Print and shaded views of the part. All mm, measured from the part's lowest x, y and z. A direction names the side the tool comes from. Coordinates: 2 decimals unless noted, no trailing zeros. Loops run counter-clockwise (first coordinate to the right, second up) from the corner with the lowest first, then second, coordinate; pieces in that order, holes last. Notation, with made-up numbers: M 45.5,59 L 68.5,59 A22 ccw 68.5,88 Z; hole C 73,-1 d8. An arc over 180 degrees is marked long. Answer as a JSON object with one key per item and string values. Group by question number.
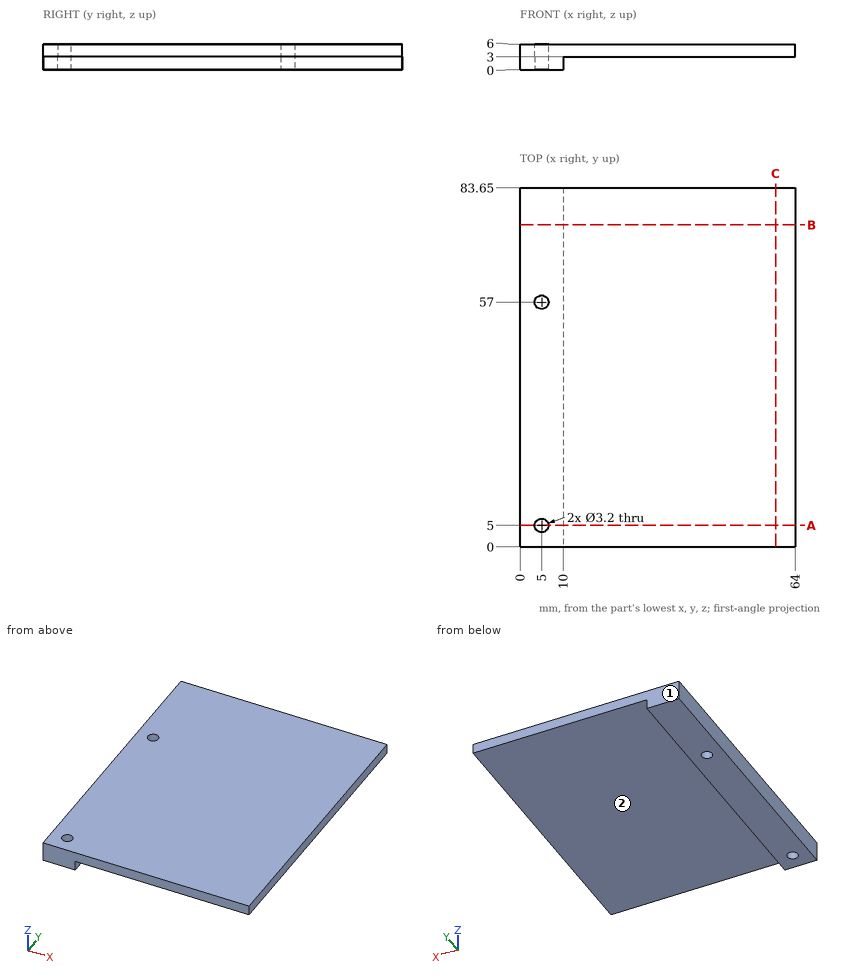
Item 1: Drill centre lines: L1, parallel to X at y = 5, z = 4.45; L2, parallel to X at y = 5, z = 1.75; L3, parallel to X at y = 77, z = 1.1. Where is each one in solid material? Low to high. Write a range as from..to.
Item 2: Slice it at B-B, the plane y = 75. Write the cut outline in (x, z).
Item 3: Pin check, flat tips, straight feed: pin 1 (2 mm diameter, centred on x = 57, y = 31.5, fed in from -Z); pin 2 (3 mm diameter, centred on y = 71.5, z = 3, fed in from -X); pin 3 (2.5 mm diameter, centred on y = 36, z = 1, fed in from +X). Stop position of each tip, or through.
Item 4: Slice it at C-C, the plane x = 59.5. Write the cut outline in (y, z).
Item 5: Slice it at A-A, the plane y = 5. Write the cut outline in (x, z).
Item 6: Tool access for the marked faces 1 and 2: list every direction of +Z, -Z, +X, -X, +Y, -Y with a clear straight run to the whole face (end or side of a thin tool).
Computed:
{
 "1": {"L1": "0..3.4, 6.6..64", "L2": "0..3.4, 6.6..10", "L3": "0..10"},
 "2": {"outline": "M 0,0 L 10,0 L 10,3 L 64,3 L 64,6 L 0,6 Z"},
 "3": {"pin 1": "z = 3", "pin 2": "x = 0", "pin 3": "x = 10"},
 "4": {"outline": "M 0,3 L 83.65,3 L 83.65,6 L 0,6 Z"},
 "5": {"outline": "M 0,0 L 3.4,0 L 3.4,6 L 0,6 Z; M 6.6,0 L 10,0 L 10,3 L 64,3 L 64,6 L 6.6,6 Z"},
 "6": {"face 1": "+Z, -Z, +X, -X, +Y", "face 2": "-Z, +X, +Y, -Y"}
}
